```python
from build123d import *

# Parameters (mm, degrees)
SKETCH_1_R          = 3
SKETCH_1_R_2        = 2
SKETCH_1_R_3        = 1.35
EXTRUDE_1_DEPTH     = 5
EXTRUDE_START       = 7
SKETCH_1_3_R        = 3
SKETCH_1_3_R_2      = 1.35
EXTRUDE_2_DEPTH     = 7
CHAMFER_1_SIZE      = 2
CHAMFER_2_SIZE      = 2
EXTRUDE_3_DEPTH     = 50
SKETCH_4_W          = 5
SKETCH_4_H          = 11.7
SKETCH_4_W_2        = 31.5
SKETCH_4_W_3        = 1.5
CUT_EXTRUDE_1_DEPTH = 12


with BuildPart() as part:
    # Sketch 1 → Extrude 1 (new body)
    # profile 1 of 9: a face of its own
    with BuildSketch(Plane(origin=(0, 0, 0), x_dir=(1, 0, 0), z_dir=(0, 1, 0))):
        with BuildLine():
            Line((3, 0), (107, 0))
            ThreePointArc((107, 0), (109.121320344, -0.878679656), (110, -3))
            Line((110, -3), (110, -157))
            ThreePointArc((110, -157), (109.121320344, -159.121320344), (107, -160))
            Line((107, -160), (3, -160))
            ThreePointArc((3, -160), (0.878679656, -159.121320344), (0, -157))
            Line((0, -157), (0, -3))
            ThreePointArc((0, -3), (0.878679656, -0.878679656), (3, 0))
        make_face()
        with Locations((43.362359308, -97.700213826)):
            Circle(SKETCH_1_R, mode=Mode.SUBTRACT)
        with Locations((10.566119403, -97.203577053)):
            Circle(SKETCH_1_R, mode=Mode.SUBTRACT)
        with Locations((98, -70)):
            Circle(SKETCH_1_R, mode=Mode.SUBTRACT)
        with Locations((40, -70)):
            Circle(SKETCH_1_R, mode=Mode.SUBTRACT)
        with Locations((40, -21)):
            Circle(SKETCH_1_R, mode=Mode.SUBTRACT)
        with Locations((98, -21)):
            Circle(SKETCH_1_R, mode=Mode.SUBTRACT)
        with Locations(Location((55, -7, 0), (0, 0, 270))):
            Circle(SKETCH_1_R_2, mode=Mode.SUBTRACT)
        with Locations(Location((55, -153, 0), (0, 0, 270))):
            Circle(SKETCH_1_R_2, mode=Mode.SUBTRACT)
        with BuildLine():
            ThreePointArc((60, -117.763932023), (59, -120), (60, -122.236067978))
            Line((60, -122.236067978), (60, -135))
            ThreePointArc((60, -135), (62, -137), (64, -135))
            Line((64, -135), (64, -122.236067978))
            ThreePointArc((64, -122.236067978), (65, -120), (64, -117.763932023))
            Line((64, -117.763932023), (64, -105))
            ThreePointArc((64, -105), (62, -103), (60, -105))
            Line((60, -105), (60, -117.763932023))
        make_face(mode=Mode.SUBTRACT)
        with BuildLine():
            ThreePointArc((96, -117.763932023), (95, -120), (96, -122.236067977))
            Line((96, -122.236067977), (96, -135))
            ThreePointArc((96, -135), (98, -137), (100, -135))
            Line((100, -135), (100, -122.236067977))
            ThreePointArc((100, -122.236067977), (101, -120), (100, -117.763932023))
            Line((100, -117.763932023), (100, -105))
            ThreePointArc((100, -105), (98, -103), (96, -105))
            Line((96, -105), (96, -117.763932023))
        make_face(mode=Mode.SUBTRACT)
    # profile 2 of 9: a face of its own
    with BuildSketch(Plane(origin=(0, 0, 0), x_dir=(1, 0, 0), z_dir=(0, 1, 0))):
        with Locations((10.566119403, -97.203577053)):
            Circle(SKETCH_1_R)
        with Locations(Location((10.566119403, -97.203577053, 0), (0, 0, 270))):
            Circle(SKETCH_1_R_3, mode=Mode.SUBTRACT)
    # profile 3 of 9: a face of its own
    with BuildSketch(Plane(origin=(0, 0, 0), x_dir=(1, 0, 0), z_dir=(0, 1, 0))):
        with Locations((40, -70)):
            Circle(SKETCH_1_R)
        with Locations(Location((40, -70, 0), (0, 0, 270))):
            Circle(SKETCH_1_R_3, mode=Mode.SUBTRACT)
    # profile 4 of 9: a face of its own
    with BuildSketch(Plane(origin=(0, 0, 0), x_dir=(1, 0, 0), z_dir=(0, 1, 0))):
        with Locations((43.362359308, -97.700213826)):
            Circle(SKETCH_1_R)
        with Locations(Location((43.362359308, -97.700213826, 0), (0, 0, 270))):
            Circle(SKETCH_1_R_3, mode=Mode.SUBTRACT)
    # profile 5 of 9: a face of its own
    with BuildSketch(Plane(origin=(0, 0, 0), x_dir=(1, 0, 0), z_dir=(0, 1, 0))):
        with BuildLine():
            Line((60, -105), (60, -117.763932023))
            ThreePointArc((60, -117.763932023), (59, -120), (60, -122.236067978))
            Line((60, -122.236067978), (60, -135))
            ThreePointArc((60, -135), (62, -137), (64, -135))
            Line((64, -135), (64, -122.236067978))
            ThreePointArc((64, -122.236067978), (65, -120), (64, -117.763932023))
            Line((64, -117.763932023), (64, -105))
            ThreePointArc((64, -105), (62, -103), (60, -105))
        make_face()
        with Locations(Location((62, -120, 0), (0, 0, 270))):
            Circle(SKETCH_1_R_3, mode=Mode.SUBTRACT)
    # profile 6 of 9: a face of its own
    with BuildSketch(Plane(origin=(0, 0, 0), x_dir=(1, 0, 0), z_dir=(0, 1, 0))):
        with BuildLine():
            Line((96, -105), (96, -117.763932023))
            ThreePointArc((96, -117.763932023), (95, -120), (96, -122.236067977))
            Line((96, -122.236067977), (96, -135))
            ThreePointArc((96, -135), (98, -137), (100, -135))
            Line((100, -135), (100, -122.236067977))
            ThreePointArc((100, -122.236067977), (101, -120), (100, -117.763932023))
            Line((100, -117.763932023), (100, -105))
            ThreePointArc((100, -105), (98, -103), (96, -105))
        make_face()
        with Locations(Location((98, -120, 0), (0, 0, 270))):
            Circle(SKETCH_1_R_3, mode=Mode.SUBTRACT)
    # profile 7 of 9: a face of its own
    with BuildSketch(Plane(origin=(0, 0, 0), x_dir=(1, 0, 0), z_dir=(0, 1, 0))):
        with Locations((98, -70)):
            Circle(SKETCH_1_R)
        with Locations(Location((98, -70, 0), (0, 0, 270))):
            Circle(SKETCH_1_R_3, mode=Mode.SUBTRACT)
    # profile 8 of 9: a face of its own
    with BuildSketch(Plane(origin=(0, 0, 0), x_dir=(1, 0, 0), z_dir=(0, 1, 0))):
        with Locations((98, -21)):
            Circle(SKETCH_1_R)
        with Locations(Location((98, -21, 0), (0, 0, 270))):
            Circle(SKETCH_1_R_3, mode=Mode.SUBTRACT)
    # profile 9 of 9: a face of its own
    with BuildSketch(Plane(origin=(0, 0, 0), x_dir=(1, 0, 0), z_dir=(0, 1, 0))):
        with Locations((40, -21)):
            Circle(SKETCH_1_R)
        with Locations(Location((40, -21, 0), (0, 0, 270))):
            Circle(SKETCH_1_R_3, mode=Mode.SUBTRACT)
    extrude(amount=-EXTRUDE_1_DEPTH)

    # Sketch 1_3 → Extrude 2 (add)
    # profile 1 of 8: a face of its own
    with BuildSketch(Plane(origin=(0, 0, 0), x_dir=(1, 0, 0), z_dir=(0, 1, 0)).offset(EXTRUDE_START)):
        with Locations(Location((40, -21, 0), (0, 0, 270))):
            Circle(SKETCH_1_3_R)
        with Locations(Location((40, -21, 0), (0, 0, 270))):
            Circle(SKETCH_1_3_R_2, mode=Mode.SUBTRACT)
    # profile 2 of 8: a face of its own
    with BuildSketch(Plane(origin=(0, 0, 0), x_dir=(1, 0, 0), z_dir=(0, 1, 0)).offset(EXTRUDE_START)):
        with Locations(Location((98, -21, 0), (0, 0, 270))):
            Circle(SKETCH_1_3_R)
        with Locations(Location((98, -21, 0), (0, 0, 270))):
            Circle(SKETCH_1_3_R_2, mode=Mode.SUBTRACT)
    # profile 3 of 8: a face of its own
    with BuildSketch(Plane(origin=(0, 0, 0), x_dir=(1, 0, 0), z_dir=(0, 1, 0)).offset(EXTRUDE_START)):
        with Locations(Location((98, -70, 0), (0, 0, 270))):
            Circle(SKETCH_1_3_R)
        with Locations(Location((98, -70, 0), (0, 0, 270))):
            Circle(SKETCH_1_3_R_2, mode=Mode.SUBTRACT)
    # profile 4 of 8: a face of its own
    with BuildSketch(Plane(origin=(0, 0, 0), x_dir=(1, 0, 0), z_dir=(0, 1, 0)).offset(EXTRUDE_START)):
        with Locations(Location((40, -70, 0), (0, 0, 270))):
            Circle(SKETCH_1_3_R)
        with Locations(Location((40, -70, 0), (0, 0, 270))):
            Circle(SKETCH_1_3_R_2, mode=Mode.SUBTRACT)
    # profile 5 of 8: a face of its own
    with BuildSketch(Plane(origin=(0, 0, 0), x_dir=(1, 0, 0), z_dir=(0, 1, 0)).offset(EXTRUDE_START)):
        with Locations(Location((43.362359308, -97.700213826, 0), (0, 0, 270))):
            Circle(SKETCH_1_3_R)
        with Locations(Location((43.362359308, -97.700213826, 0), (0, 0, 270))):
            Circle(SKETCH_1_3_R_2, mode=Mode.SUBTRACT)
    # profile 6 of 8: a face of its own
    with BuildSketch(Plane(origin=(0, 0, 0), x_dir=(1, 0, 0), z_dir=(0, 1, 0)).offset(EXTRUDE_START)):
        with Locations(Location((10.566119403, -97.203577053, 0), (0, 0, 270))):
            Circle(SKETCH_1_3_R)
        with Locations(Location((10.566119403, -97.203577053, 0), (0, 0, 270))):
            Circle(SKETCH_1_3_R_2, mode=Mode.SUBTRACT)
    # profile 7 of 8: a face of its own
    with BuildSketch(Plane(origin=(0, 0, 0), x_dir=(1, 0, 0), z_dir=(0, 1, 0)).offset(EXTRUDE_START)):
        with BuildLine():
            Line((60, -105), (60, -117.763932023))
            ThreePointArc((60, -117.763932023), (59, -120), (60, -122.236067978))
            Line((60, -122.236067978), (60, -135))
            ThreePointArc((60, -135), (62, -137), (64, -135))
            Line((64, -135), (64, -122.236067978))
            ThreePointArc((64, -122.236067978), (65, -120), (64, -117.763932023))
            Line((64, -117.763932023), (64, -105))
            ThreePointArc((64, -105), (62, -103), (60, -105))
        make_face()
        with Locations(Location((62, -120, 0), (0, 0, 270))):
            Circle(SKETCH_1_3_R_2, mode=Mode.SUBTRACT)
    # profile 8 of 8: a face of its own
    with BuildSketch(Plane(origin=(0, 0, 0), x_dir=(1, 0, 0), z_dir=(0, 1, 0)).offset(EXTRUDE_START)):
        with BuildLine():
            Line((96, -105), (96, -117.763932023))
            ThreePointArc((96, -117.763932023), (95, -120), (96, -122.236067977))
            Line((96, -122.236067977), (96, -135))
            ThreePointArc((96, -135), (98, -137), (100, -135))
            Line((100, -135), (100, -122.236067977))
            ThreePointArc((100, -122.236067977), (101, -120), (100, -117.763932023))
            Line((100, -117.763932023), (100, -105))
            ThreePointArc((100, -105), (98, -103), (96, -105))
        make_face()
        with Locations(Location((98, -120, 0), (0, 0, 270))):
            Circle(SKETCH_1_3_R_2, mode=Mode.SUBTRACT)
    extrude(amount=-EXTRUDE_2_DEPTH)

    # Chamfer 1
    chamfer_1_edges = [part.edges().sort_by_distance(p)[0] for p in [
        (55, 0, 5),
    ]]
    chamfer(chamfer_1_edges, length=CHAMFER_1_SIZE)

    # Chamfer 2
    chamfer_2_edges = [part.edges().sort_by_distance(p)[0] for p in [
        (55, 0, 151),
    ]]
    chamfer(chamfer_2_edges, length=CHAMFER_2_SIZE)

    # Sketch 3 → Extrude 3 (add)
    with BuildSketch(Plane.ZY):
        Polygon((142.5, 0), (142.5, 7), (145.5, 7), (145.5, 8.7), (142.5, 8.7), (142.5, 10.2), (144, 11.7), (148.5, 11.7), (148.5, 0), align=None)
    extrude(amount=-EXTRUDE_3_DEPTH)

    # Sketch 4 → Cut-Extrude 1 (cut)
    with BuildSketch(Plane.XY.offset(148.5)):
        with Locations((2.5, 5.85)):
            Rectangle(SKETCH_4_W, SKETCH_4_H)
        with Locations((26.75, 5.85)):
            Rectangle(SKETCH_4_W_2, SKETCH_4_H)
        with Locations((49.25, 5.85)):
            Rectangle(SKETCH_4_W_3, SKETCH_4_H)
    extrude(amount=-CUT_EXTRUDE_1_DEPTH, mode=Mode.SUBTRACT)


solid = part.part
```
Geometry check sheet. Reference: the model listing, model coordinates, mm. A direction names the side the tool comes from. Coordinates: 2 decimals unless noted, no trailing zeros. Write each loop counter-clockwise with the first axis right and the second up, starting at its lowest first coordinate (ties: lowest second). Pieces come first, ordered by that corner, then holes. Notation, with made-up numbers: (15.25, 53.25) -> (60.25, 53.25) arc R24 cw to (60.25, 92.25) -> close; hole circle Ø3 at (60.25, -34). An arc over 180 degrees is marked (long way). Use CSV: the item, a comma, the result in double quotes. Start each with the question number.
Item 1: Mould release check, pull along Y, two halves, no side actions. Record for faces 5 (the flat face through (100, 4, 111)), 6 (the flat face through (8, 8.7, 144)), 7 (the flat face through (8, 11.7, 146)): released by +Y, released by -Y, zero draft, split by the parting line, or undercut.
Item 2: Set-up check for faces 1 (the flat face through (8, 3, 142.5)), 2 (the flat face through (45, 7, 144)), 3 (the cylindrical face through (44.263, 3.549, 100.562)), 4 (the flat face through (45, 6, 148.5)): record each of +Z, -Z, +X, -X, +Y, -Y from which the full face is reachable in a straight line by a thin tool's end or side.
Item 3: Cross-section at A-A, the plane z = 7. Record the cut outline in (x, y).
Item 4: Thickness scan on line 1 (X direction, y = 0.5, z = 70); line 2 (X direction, y = -1, z = 21); line 3 (Z direction, x = 98, y = -1.5). Record the ranges inside material, lowest first.
Item 5: Depth check by flat-ended pin: pin 1 Ø5 at (x, z) = (55, 7) entering from +Y; pin 2 Ø3 at (x, z) = (98, 71) entering from +Y; pin 3 Ø0.8 at (x, y) = (46.5, 8) entering from -Z. Enter the tip coordinate at first touch or a pass-through.
Item 6: Cross-section at C-C, the plane z = 81. Record the cut outline in (x, y).
Item 7: Cross-section at B-B, the plane x = 19. Record the cut outline in (y, z).
Answers:
1,face 5,"zero draft"
1,face 6,"undercut"
1,face 7,"released by +Y"
2,face 1,"+X, -X, +Y"
2,face 2,"-Z, +X, -X"
2,face 3,"+Y"
2,face 4,"+Z, +X, -X, +Y"
3,outline,"(0, -5) -> (53, -5) -> (53, -2) -> (51, 0) -> (0, 0) -> close; (57, -5) -> (110, -5) -> (110, 0) -> (59, 0) -> (57, -2) -> close"
4,line 1,"37 to 38.65, 41.35 to 43, 95 to 96.65, 99.35 to 101"
4,line 2,"0 to 38.65, 41.35 to 96.65, 99.35 to 110"
4,line 3,"0 to 19.65, 22.35 to 68.65, 71.35 to 118.65, 121.35 to 160"
5,pin 1,"y = -1.5"
5,pin 2,"y = 7"
5,pin 3,"z = 145.5"
6,outline,"(0, -5) -> (110, -5) -> (110, 0) -> (0, 0) -> close"
7,outline,"(-5, 0) -> (0, 0) -> (0, 160) -> (-5, 160) -> close"
